from build123d import *

# Parameters (mm, degrees)
MAINBODY_DEPTH                 = 10
SCREWCUTOUTS_DEPTH             = 197.85019685
SKETCH3_R                      = 4
SKETCH3_R_2                    = 1.55
RODCUTOUTS_DEPTH               = 197.85019685
SKETCH6_R                      = 1.55
CUT_EXTRUDE1_DEPTH             = 197.85019685
BEDADJUSTMENTSCREWCUTOUT_DEPTH = 197.85019685
DIRECTIONKEY_DEPTH             = 197.85019685
CUT_EXTRUDE2_DEPTH             = 197.85019685


with BuildPart() as part:
    # Sketch1 → MainBody (new body)
    with BuildSketch(Plane(origin=(0, 0, 0), x_dir=(1, 0, 0), z_dir=(0, 1, 0))):
        Polygon((0, 25), (0, -25), (-185, -25), (-185, -9), (-195, -9), (-195, 1), (-185, 1), (-185, 25), align=None)
    mainbody = extrude(amount=MAINBODY_DEPTH)

    # Sketch5 → ScrewCutouts (cut, through all)
    with BuildSketch(Plane(origin=(0, 10, 0), x_dir=(1, 0, 0), z_dir=(0, 1, 0))):
        with BuildLine():
            Line((-185, 9.75), (-181.2, 9.75))
            Line((-181.2, 9.75), (-181.2, 10.75))
            ThreePointArc((-181.2, 10.75), (-181.126776695, 10.926776695), (-180.95, 11))
            Line((-180.95, 11), (-177.25, 11))
            ThreePointArc((-177.25, 11), (-177.073223305, 10.926776695), (-177, 10.75))
            Line((-177, 10.75), (-177, 9.75))
            Line((-177, 9.75), (-174.5, 9.75))
            Line((-174.5, 9.75), (-174.5, 6.25))
            Line((-174.5, 6.25), (-177, 6.25))
            Line((-177, 6.25), (-177, 5.25))
            ThreePointArc((-177, 5.25), (-177.073223305, 5.073223305), (-177.25, 5))
            Line((-177.25, 5), (-180.95, 5))
            ThreePointArc((-180.95, 5), (-181.126776695, 5.073223305), (-181.2, 5.25))
            Line((-181.2, 5.25), (-181.2, 6.25))
            Line((-181.2, 6.25), (-185, 6.25))
            Line((-185, 6.25), (-185, 9.75))
        make_face()
        with BuildLine():
            Line((-185, -14.25), (-181.2, -14.25))
            Line((-181.2, -14.25), (-181.2, -13.25))
            ThreePointArc((-181.2, -13.25), (-181.126776695, -13.073223305), (-180.95, -13))
            Line((-180.95, -13), (-177.25, -13))
            ThreePointArc((-177.25, -13), (-177.073223305, -13.073223305), (-177, -13.25))
            Line((-177, -13.25), (-177, -14.25))
            Line((-177, -14.25), (-174.5, -14.25))
            Line((-174.5, -14.25), (-174.5, -17.75))
            Line((-174.5, -17.75), (-177, -17.75))
            Line((-177, -17.75), (-177, -18.75))
            ThreePointArc((-177, -18.75), (-177.073223305, -18.926776695), (-177.25, -19))
            Line((-177.25, -19), (-180.95, -19))
            ThreePointArc((-180.95, -19), (-181.126776695, -18.926776695), (-181.2, -18.75))
            Line((-181.2, -18.75), (-181.2, -17.75))
            Line((-181.2, -17.75), (-185, -17.75))
            Line((-185, -17.75), (-185, -14.25))
        make_face()
    screwcutouts = extrude(amount=-SCREWCUTOUTS_DEPTH, mode=Mode.SUBTRACT)

    # Mirror1: MainBody, ScrewCutouts across plane
    add(mainbody.mirror(Plane(origin=(0, 0, 0), x_dir=(0, 0, 1), z_dir=(1, 0, 0))))
    add(screwcutouts.mirror(Plane(origin=(0, 0, 0), x_dir=(0, 0, 1), z_dir=(1, 0, 0))), mode=Mode.SUBTRACT)

    # Sketch3 → RodCutouts (cut, through all)
    with BuildSketch(Plane(origin=(0, 10, 0), x_dir=(1, 0, 0), z_dir=(0, 1, 0))):
        with Locations((-73, 21.5)):
            Circle(SKETCH3_R)
        with Locations(Location((-83, 20.5, 0), (0, 0, 270))):
            Circle(SKETCH3_R_2)
        with Locations(Location((-63, 20.5, 0), (0, 0, 90))):
            Circle(SKETCH3_R_2)
        with Locations(Location((67, 20.5, 0), (0, 0, 270))):
            Circle(SKETCH3_R_2)
        with Locations(Location((87, 20.5, 0), (0, 0, 90))):
            Circle(SKETCH3_R_2)
        with Locations((77, 21.5)):
            Circle(SKETCH3_R)
    extrude(amount=-RODCUTOUTS_DEPTH, mode=Mode.SUBTRACT)

    # Sketch6 → Cut-Extrude1 (cut, through all)
    with BuildSketch(Plane(origin=(0, 10, 0), x_dir=(1, 0, 0), z_dir=(0, 1, 0))):
        with Locations(Location((-13, 4, 0), (0, 0, 270))):
            Circle(SKETCH6_R)
        with Locations(Location((17, 4, 0), (0, 0, 90))):
            Circle(SKETCH6_R)
    extrude(amount=-CUT_EXTRUDE1_DEPTH, mode=Mode.SUBTRACT)

    # Sketch7 → BedAdjustmentScrewCutout (cut, through all)
    with BuildSketch(Plane(origin=(0, 10, 0), x_dir=(1, 0, 0), z_dir=(0, 1, 0))):
        with BuildLine():
            Line((-98.5, 25), (-98.5, 23))
            ThreePointArc((-98.5, 23), (-102.5, 19), (-106.5, 23))
            Line((-106.5, 23), (-106.5, 25))
            ThreePointArc((-106.5, 25), (-102.5, 29), (-98.5, 25))
        make_face()
        with BuildLine():
            Line((102.5, 25), (102.5, 23))
            ThreePointArc((102.5, 23), (106.5, 19), (110.5, 23))
            Line((110.5, 23), (110.5, 25))
            ThreePointArc((110.5, 25), (106.5, 29), (102.5, 25))
        make_face()
    extrude(amount=-BEDADJUSTMENTSCREWCUTOUT_DEPTH, mode=Mode.SUBTRACT)

    # Sketch8 → DirectionKey (cut, through all)
    with BuildSketch(Plane(origin=(0, 10, 0), x_dir=(1, 0, 0), z_dir=(0, 1, 0))):
        Polygon((88.35, 20.5), (89.35, 21.5), (89.35, 19.5), align=None)
    extrude(amount=-DIRECTIONKEY_DEPTH, mode=Mode.SUBTRACT)

    # Sketch9 → Cut-Extrude2 (cut, through all)
    with BuildSketch(Plane(origin=(0, 10, 0), x_dir=(1, 0, 0), z_dir=(0, 1, 0))):
        with BuildLine():
            Line((6, 27), (6, 23))
            ThreePointArc((6, 23), (2, 19), (-2, 23))
            Line((-2, 23), (-2, 27))
            ThreePointArc((-2, 27), (2, 31), (6, 27))
        make_face()
    extrude(amount=-CUT_EXTRUDE2_DEPTH, mode=Mode.SUBTRACT)


solid = part.part
Design review of the part built by this model. Coordinates are the model's own, in mm. A direction names the side the tool comes from. Coordinates: 2 decimals unless noted, no trailing zeros. Order: outer loops, then holes, each group sorted by start corner. A loop starts at its lowest first (then second) coordinate and runs counter-clockwise, first axis right, second up. Notation, with made-up numbers: (-38.5, 12.25) -> (-15.5, 12.25) arc R27 cw to (-15.5, 28.25) -> close; hole circle Ø11 at (23, 65). An arc over 180 degrees is marked (long way). Use one line per item in the form item = value. Start each with the question number.
(1) Add section B-B on x = -102.5. State the section outline as (y, z) points.
(2) Add section A-A on y = 5.75. Give the number of separate pieces and of enclosed holes in the cut face, plus the area to 3 significant figures.
(3) For probe 1 along X at (y, z) = (2, -4); probe 2 along X at (y, z) = (4.25, -18); probe 3 along Z at (x, y) = (175.5, 3.5), list the stretches that pass through material, from the lowest coordinate up.
(4) The part is to be moulded in two halves that separate along X. For faces 5 (the flat face through (185, 5, 21)), 6 (the cylindrical face through (2, 5, -19)), 7 (the cylindrical face through (106.4, 5.1, -19)), 8 (the flat face through (-145, 5, -25)), say which applies: +X half, -X half, draft (parallel to the pull), parting line (faces both ways), or undercut.
(5) Insertion check: pin 1 (5 mm diameter, centred on x = 77, z = -21.5, fed in from -Y); pin 2 (0.5 mm diameter, centred on y = 5, z = -6, fed in from +X); pin 3 (1.1 mm diameter, centred on y = 4, z = -5.5, fed in from -X); pin 4 (6 mm diameter, centred on x = 55, z = 8.5, fed in from -Y). Each pin has a flat end and moves straight along its axis. Give the tip position at first contact, or say it passes through.
(6) For faces 1 (the flat face through (-185, 5, -17)), 2 (the flat face through (-190, 5, 9)), 3 (the flat face through (190, 5, 9)), 4 (the flat face through (185, 5, -17)), list the 3-axis set-ups (+Z, -Z, +X, -X, +Y, -Y) from which the entire face can be reached by the end or side of a thin tool; tool diameter is ignored.
Answer block:
q1.outline = (0, -19) -> (10, -19) -> (10, 25) -> (0, 25) -> close
q2.separate_pieces = 1
q2.enclosed_holes = 6
q2.area = 18,200 mm²
q3.probe_1 = -185 to -14.55, -11.45 to 15.45, 18.55 to 185
q3.probe_2 = -185 to -74.94, -71.06 to 75.06, 78.94 to 185
q3.probe_3 = -25 to -9.75, -6.25 to 14.25, 17.75 to 25
q4.face_5 = +X half
q4.face_6 = undercut
q4.face_7 = undercut
q4.face_8 = draft
q5.pin_1 = through
q5.pin_2 = 185
q5.pin_3 = -185
q5.pin_4 = 0
q6.face_1 = -Z, -X, +Y, -Y
q6.face_2 = +Z, -X, +Y, -Y
q6.face_3 = +Z, +X, +Y, -Y
q6.face_4 = -Z, +X, +Y, -Y
